Print and shaded views of the part. All mm, measured from the part's lowest x, y and z. A direction names the side the tool comes from. Round coordinates to 2 decimals unless told otherwise and drop trailing zeros. Loops run counter-clockwise (first coordinate to the right, second up) from the corner with the lowest first, then second, coordinate; pieces in that order, holes last. Notation, with made-up numbers: (-5, 13.25) -> (48, 13.25) arc R24 ccw to (48, 32.25) -> close; hole circle Ø4 at (85, -32). An arc over 180 degrees is marked (long way). Use a Markdown table: item, result.
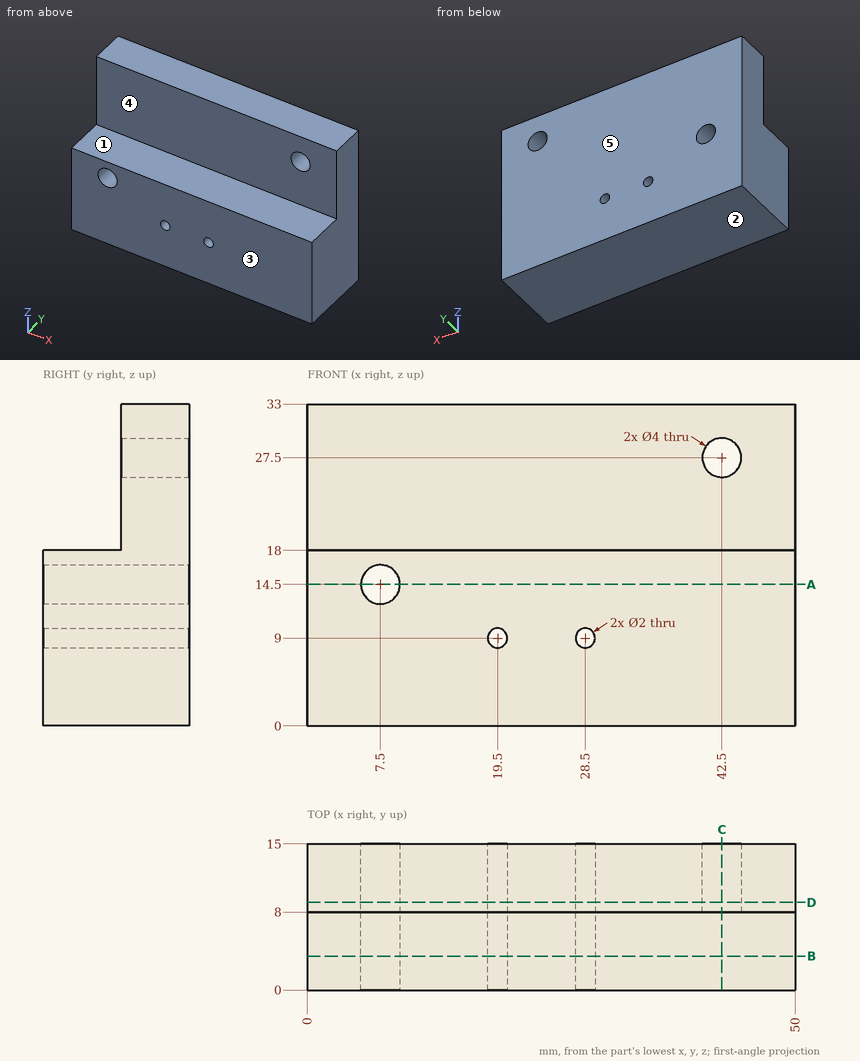
Q1. Band-saw the part on A-A, the plane z = 14.5. Give the cut face in (x, y).
Results list:
| item | result |
|---|---|
| outline | (0, 0) -> (5.5, 0) -> (5.5, 15) -> (0, 15) -> close; (9.5, 0) -> (50, 0) -> (50, 15) -> (9.5, 15) -> close |
Q2. Tool access for the marked faces 4 and 5: list every direction of +Z, -Z, +X, -X, +Y, -Y with a clear straight run to the whole face (end or side of a thin tool).
Results list:
| item | result |
|---|---|
| face 4 | +Z, +X, -X, -Y |
| face 5 | +Z, -Z, +X, -X, +Y |
Q3. Band-saw the part on D-D, the plane y = 9. Give the cut face in (x, z).
Results list:
| item | result |
|---|---|
| outline | (0, 0) -> (50, 0) -> (50, 33) -> (0, 33) -> close; hole circle Ø4 at (7.5, 14.5); hole circle Ø2 at (19.5, 9); hole circle Ø2 at (28.5, 9); hole circle Ø4 at (42.5, 27.5) |
Q4. Band-saw the part on B-B, the plane y = 3.5. Give the cut face in (x, z).
Results list:
| item | result |
|---|---|
| outline | (0, 0) -> (50, 0) -> (50, 18) -> (0, 18) -> close; hole circle Ø4 at (7.5, 14.5); hole circle Ø2 at (19.5, 9); hole circle Ø2 at (28.5, 9) |
Q5. Band-saw the part on C-C, the plane x = 42.5. Give the cut face in (y, z).
Results list:
| item | result |
|---|---|
| outline | (0, 0) -> (15, 0) -> (15, 25.5) -> (8, 25.5) -> (8, 18) -> (0, 18) -> close; (8, 29.5) -> (15, 29.5) -> (15, 33) -> (8, 33) -> close |
Q6. Pull direction Z, two halves, no side cores. Call the marked faces 1, 2 and 3: released by +Z, released by -Z, zero draft, split by the parting line, or undercut.
Results list:
| item | result |
|---|---|
| face 1 | released by +Z |
| face 2 | released by -Z |
| face 3 | zero draft |
Q7. Flat gauge pins, fed straight in: pin 1 (1.5 mm diameter, centred on x = 34, y = 2.5, fed in from -Z); pin 2 (1.2 mm diameter, centred on x = 28.5, z = 9, fed in from +Y); pin 3 (3 mm diameter, centred on x = 34.5, z = 24.5, fed in from -Y); pin 4 (2 mm diameter, centred on x = 22.5, y = 4, fed in from +Z). Where does each tip first touch, or does it go through?
Results list:
| item | result |
|---|---|
| pin 1 | stops at z = 0 |
| pin 2 | passes through |
| pin 3 | stops at y = 8 |
| pin 4 | stops at z = 18 |
Q8. Drill centre lines: L1, parallel to Z at x = 19.5, y = 11.5; L2, parallel to Z at x = 7.5, y = 10.25; L3, parallel to Z at x = 43, y = 2.75. Where is each one in solid material? Low to high. Write a range as from..to.
Results list:
| item | result |
|---|---|
| L1 | z = 0..8, 10..33 |
| L2 | z = 0..12.5, 16.5..33 |
| L3 | z = 0..18 |
